Read the model definition and answer for the solid it produces. Units are mm, in the model's axes. A direction names the side the tool comes from. Give positions to 0.01 mm unless a question says otherwise; leave off trailing zeros. Order: outer loops, then holes, each group sorted by start corner. A loop starts at its lowest first (then second) coordinate and runs counter-clockwise, first axis right, second up.
```python
from build123d import *

# Parameters (mm, degrees)
ESQUISSE1_R             = 1.5
BOSS_EXTRU_1_DEPTH      = 15
BOSS_EXTRU_2_DEPTH      = 6
BOSS_EXTRU_2_DEPTH_BACK = 1
ESQUISSE2_R             = 1.5


with BuildPart() as part:
    # Esquisse1 → Boss.-Extru.1 (new body)
    with BuildSketch(Plane(origin=(0, 0, 0), x_dir=(1, 0, 0), z_dir=(0, 1, 0))):
        Polygon((1.58771324, 2.75), (-1.58771324, 2.75), (-3.175426481, 0), (-1.58771324, -2.75), (1.58771324, -2.75), (3.175426481, 0), align=None)
        with Locations(Location((0, 0, 0), (0, 0, 270))):
            Circle(ESQUISSE1_R, mode=Mode.SUBTRACT)
    extrude(amount=BOSS_EXTRU_1_DEPTH)

    # Esquisse2 → Boss.-Extru.2 (add, two sides: drawn at the far end of the back side and taken through both)
    with BuildSketch(Plane.XZ.offset(-BOSS_EXTRU_2_DEPTH_BACK)):
        with Locations(Location((0, 0, 0), (0, 0, 270))):
            Circle(ESQUISSE2_R)
    extrude(amount=BOSS_EXTRU_2_DEPTH + BOSS_EXTRU_2_DEPTH_BACK)


solid = part.part
```
1) Consider L1, parallel to Z at x = 0, y = 11; L2, parallel to Y at x = 0.5, z = -1.1; L3, parallel to Y at x = 1.5, z = -2.1. Determine where each line is inside the solid, lowest interval first.
Final values:
L1: z = -2.75 to -1.5, 1.5 to 2.75
L2: y = -6 to 1
L3: y = 0 to 15
2) The part is cut by section C-C on z = -0.5. Determine the outline of the cut face in (x, y), and give its area (3 significant figures).
Final values:
outline: (-2.89, 0) - (-1.41, 0) - (-1.41, -6) - (1.41, -6) - (1.41, 0) - (2.89, 0) - (2.89, 15) - (1.41, 15) - (1.41, 1) - (-1.41, 1) - (-1.41, 15) - (-2.89, 15) - close
area: 64.0 mm2
3) For a pull along Z with two mould halves and no side action, classify faces 1 (the face through (1.4, 15, -1.3)), 2 (the face through (0, 1, 0)), 3 (the face through (0, 7, 2.75)), 4 (the face through (-2.37, 7.395, -1.394)) as released by +Z, released by -Z, zero draft, split by the parting line, or undercut.
Final values:
face 1: zero draft
face 2: undercut
face 3: released by +Z
face 4: released by -Z
4) A tool of negligible diameter and unlimited length cuts with its end or side. For faces 5 (the face through (0.45, 7.9, 1.43)), 6 (the face through (2.37, 7.395, 1.394)), 7 (the face through (1.4, 0, -1.3)), from which of +Z, -Z, +X, -X, +Y, -Y can it reach the whole face along a straight path? Write none if from no direction.
Final values:
face 5: +Y
face 6: +Z, +X, +Y, -Y
face 7: -Y
5) The part is cut by section B-B on x = 0. Determine the outline of the cut face in (y, z).
Final values:
outline: (-6, -1.5) - (0, -1.5) - (0, -2.75) - (15, -2.75) - (15, -1.5) - (1, -1.5) - (1, 1.5) - (15, 1.5) - (15, 2.75) - (0, 2.75) - (0, 1.5) - (-6, 1.5) - close
6) The part is cut by section A-A on y = 12.5. Determine the outline of the cut face in (x, z), and give its area (3 significant figures).
Final values:
outline: (-3.18, 0) - (-1.59, -2.75) - (1.59, -2.75) - (3.18, 0) - (1.59, 2.75) - (-1.59, 2.75) - close; hole circle Ø3 at (0, 0)
area: 19.1 mm2
7) Given pin 1 (2.5 mm diameter, centred on x = 0, z = -0.5, fed in from +Y); pin 2 (1.5 mm diameter, centred on x = 2.5, z = -0.5, fed in from -Y), each flat-ended and moving along its own axis, determine where each tip first touches the part or whether it passes through.
Final values:
pin 1: stops at y = 15
pin 2: stops at y = 0
8) The part is cut by section D-D on y = -2.75. Determine the outline of the cut face in (x, z).
Final values:
outline: circle Ø3 at (0, 0)
